Study the drawing (mm; zero at the part's minimum x, y, z) and answer. A direction names the side the tool comes from. Coordinates: 2 decimals unless noted, no trailing zeros. Write each loop counter-clockwise with the first axis right and the second up, starting at its lowest first coordinate (ties: lowest second). Pieces come first, ordered by that corner, then holes. Notation, with made-up numbers: (28.5, -4.5) - (36.5, -4.5) arc R15 cw to (36.5, 3.5) - close; hole circle Ø10 at (-22.75, -19). An arc over 180 degrees is marked (long way). One line per item, written item: value.
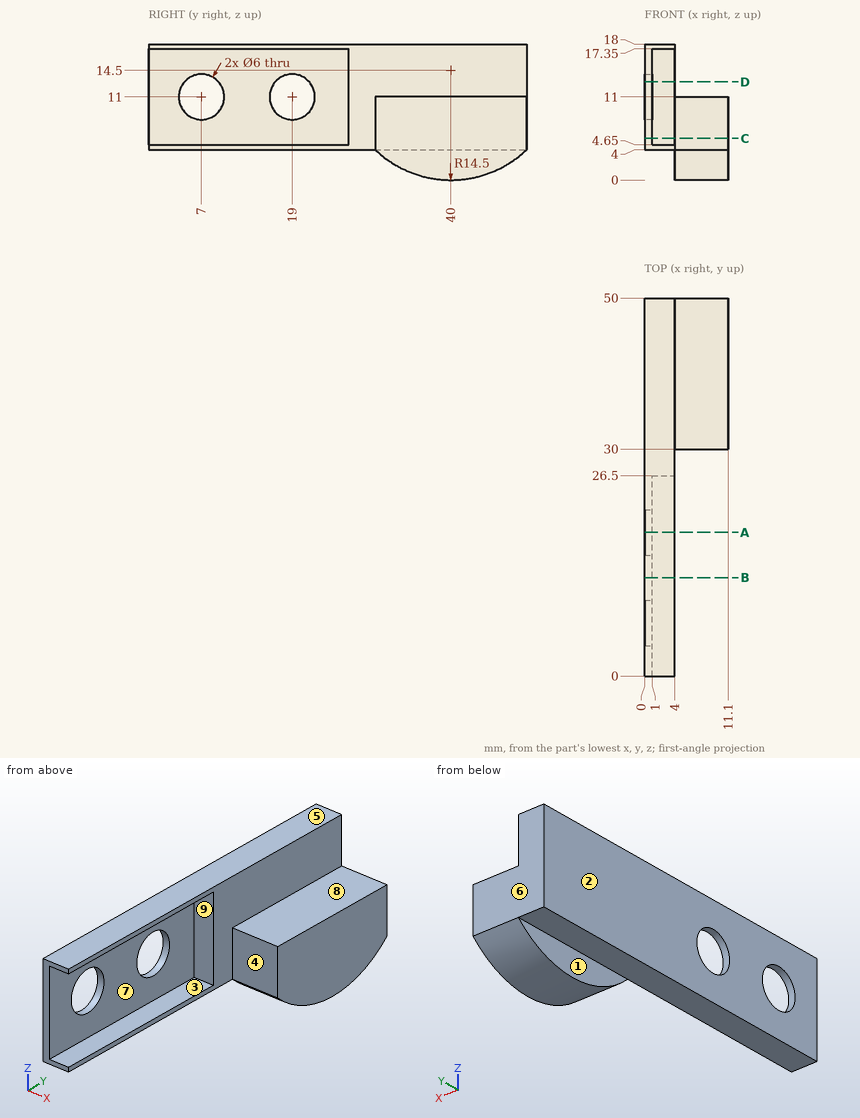
Item 1: Section C-C, the plane z = 5.5 is taken. Determine the outline of the cut face in (x, y).
Evaluation:
outline: (0, 0) - (1, 0) - (1, 26.5) - (4, 26.5) - (4, 30) - (11.1, 30) - (11.1, 50) - (0, 50) - close
Item 2: Given pin 1 (3.5 mm diameter, centred on x = 2, y = 9.5, fed in from -Z); pin 2 (0.9 mm diameter, centred on x = 2, z = 10, fed in from -Y); pin 3 (4 mm diameter, centred on y = 13, z = 10.5, fed in from +X), each flat-ended and moving along its own axis, determine where each tip first touches the part or whether it passes through.
Evaluation:
pin 1: stops at z = 4
pin 2: stops at y = 26.5
pin 3: stops at x = 1
Item 3: Section D-D, the plane z = 13 is taken. Determine the outline of the cut face in (x, y).
Evaluation:
outline: (0, 0) - (1, 0) - (1, 4.76) - (0, 4.76) - close; (0, 9.24) - (1, 9.24) - (1, 16.76) - (0, 16.76) - close; (0, 21.24) - (1, 21.24) - (1, 26.5) - (4, 26.5) - (4, 50) - (0, 50) - close
Item 4: Determine the mould class of the marked faces 6, 7, 8 and 9 for opening direction Z: +Z half, -Z half, draft (parallel to the pull), parting line (faces both ways), or undercut.
Evaluation:
face 6: draft
face 7: undercut
face 8: +Z half
face 9: undercut
Item 5: Section B-B, the plane y = 13 is taken. Determine the outline of the cut face in (x, z), then the cut area to 3 significant figures.
Evaluation:
outline: (0, 4) - (4, 4) - (4, 4.65) - (1, 4.65) - (1, 17.35) - (4, 17.35) - (4, 18) - (0, 18) - close
area: 17.9 mm2
Item 6: Which of the six approach directions +Z, -Z, +X, -X, +Y, -Y give full straight-line access (tool end or side, diameter ignored) to the marked faces 1, 2, 3, 4 and 5?
Evaluation:
face 1: -Z, -X, +Y, -Y
face 2: +Z, -Z, -X, +Y, -Y
face 3: +X, -Y
face 4: +Z, -Z, +X, -Y
face 5: +Z, +X, -X, +Y, -Y
Item 7: Section A-A, the plane y = 19 is taken. Determine the outline of the cut face in (x, z), then the cut area to 3 significant figures.
Evaluation:
outline: (0, 4) - (4, 4) - (4, 4.65) - (1, 4.65) - (1, 8) - (0, 8) - close; (0, 14) - (1, 14) - (1, 17.35) - (4, 17.35) - (4, 18) - (0, 18) - close
area: 11.9 mm2
Item 8: Consider probe 1 along Y at (x, z) = (0.45, 11); probe 2 along Z at (x, y) = (1.25, 18); probe 3 along X at (y, z) = (7, 17.25). Determine where each line is inside the solid, lowest interval first.
Evaluation:
probe 1: y = 0 to 4, 10 to 16, 22 to 50
probe 2: z = 4 to 4.65, 17.35 to 18
probe 3: x = 0 to 1
